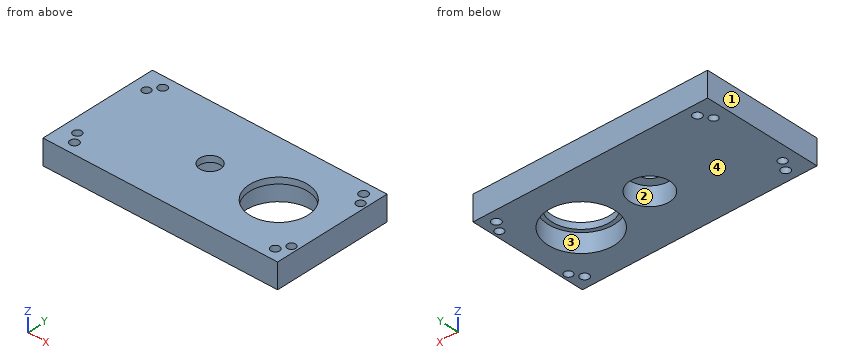
```python
from build123d import *

# Parameters (mm, degrees)
ESBO_O1_W                = 118
ESBO_O1_H                = 62
ESBO_O1_R                = 9.5
ESBO_O1_R_2              = 16
ESBO_O1_R_3              = 2
RESSALTO_EXTRUS_O1_DEPTH = 12
FURO_COM_FOLGA_DE_M51_D  = 4.2
RESSALTO_EXTRUS_O4_START = -3
ESBO_O17_R               = 9.5
RESSALTO_EXTRUS_O4_DEPTH = 3
ESBO_O18_W               = 118
ESBO_O18_H               = 62
ESBO_O18_W_2             = 112.82
ESBO_O18_H_2             = 57
CORTE_EXTRUS_O3_DEPTH    = 68.720011813
RESSALTO_EXTRUS_O5_START = -3
ESBO_O19_R               = 16
ESBO_O19_R_2             = 14
RESSALTO_EXTRUS_O5_DEPTH = 3
ESBO_O21_R               = 5
CORTE_EXTRUS_O4_DEPTH    = 10


with BuildPart() as part:
    # Esboço1 → Ressalto-extrusão1 (new body)
    with BuildSketch(Plane.XY):
        Rectangle(ESBO_O1_W, ESBO_O1_H)
        with Locations((-4.25, 0)):
            Circle(ESBO_O1_R, mode=Mode.SUBTRACT)
        with Locations((28.75, 0)):
            Circle(ESBO_O1_R_2, mode=Mode.SUBTRACT)
        with Locations((51.5, -18)):
            Circle(ESBO_O1_R_3, mode=Mode.SUBTRACT)
        with Locations((51.5, 18)):
            Circle(ESBO_O1_R_3, mode=Mode.SUBTRACT)
        with Locations((-51.5, -18)):
            Circle(ESBO_O1_R_3, mode=Mode.SUBTRACT)
        with Locations((-51.5, 18)):
            Circle(ESBO_O1_R_3, mode=Mode.SUBTRACT)
    extrude(amount=RESSALTO_EXTRUS_O1_DEPTH)

    # Furo com folga de M51 (through all)
    with Locations(Plane.XY.offset(12)):
        with Locations((-48.32, 23), (-48.32, -23), (48.32, -23), (48.32, 23)):
            Hole(FURO_COM_FOLGA_DE_M51_D / 2)

    # Esboço17 → Ressalto-extrusão4 (add)
    with BuildSketch(Plane.XY.offset(12).offset(RESSALTO_EXTRUS_O4_START)):
        with Locations((-4.25, 0)):
            Circle(ESBO_O17_R)
    extrude(amount=RESSALTO_EXTRUS_O4_DEPTH)

    # Esboço18 → Corte-extrusão3 (cut, through all)
    with BuildSketch(Plane.XY.offset(12)):
        Rectangle(ESBO_O18_W, ESBO_O18_H)
        with Locations((-1.91, 0)):
            Rectangle(ESBO_O18_W_2, ESBO_O18_H_2, mode=Mode.SUBTRACT)
    extrude(amount=-CORTE_EXTRUS_O3_DEPTH, mode=Mode.SUBTRACT)

    # Esboço19 → Ressalto-extrusão5 (add)
    with BuildSketch(Plane.XY.offset(12).offset(RESSALTO_EXTRUS_O5_START)):
        with Locations((28.75, 0)):
            Circle(ESBO_O19_R)
        with Locations((28.75, 0)):
            Circle(ESBO_O19_R_2, mode=Mode.SUBTRACT)
    extrude(amount=RESSALTO_EXTRUS_O5_DEPTH)

    # Esboço21 → Corte-extrusão4 (cut)
    with BuildSketch(Plane(origin=(0, 0, 9), x_dir=(-1, 0, 0), z_dir=(0, 0, -1))):
        with Locations((4.25, 0)):
            Circle(ESBO_O21_R)
    extrude(amount=-CORTE_EXTRUS_O4_DEPTH, mode=Mode.SUBTRACT)


solid = part.part
```
Geometry check sheet. Reference: the model listing, model coordinates, mm. Face numbers are marked on the shaded views. Coordinates: 2 decimals unless noted, no trailing zeros. Loops run counter-clockwise (first coordinate to the right, second up) from the corner with the lowest first, then second, coordinate; pieces in that order, holes last.
Item 1: Release check for a two-part mould opening along X. For the marked faces 1, 2, 3 and 4 record: released by +X, released by -X, zero draft, split by the parting line, or undercut.
Item 2: Sectioned sample at B-B, the plane y = 23. Record the boundary of the cut face in (x, z), then the cut area to 3 significant figures.
Item 3: Sectioned sample at A-A, the plane x = 51.5. Record the boundary of the cut face in (y, z), then the cut area to 3 significant figures.
Item 4: Go/stop test with a flat-tipped pin: pin 1 Ø4.5 at (x, y) = (51.5, -18) entering from -Z. Record where the tip stops, or that it passes through.
Item 5: Thickness scan on line 1 (Y direction, x = 48.32, z = 4.5); line 2 (Y direction, x = 28.75, z = 2.75); line 3 (Y direction, x = -4.25, z = 4.25). Record the ranges inside material, lowest first.
Item 6: Sectioned sample at D-D, the plane x = -4.25. Record the boundary of the cut face in (y, z).
Item 7: Sectioned sample at C-C, the plane z = 6. Count the separate pieces of the cut face and the enclosed holes in it, then the cut area to 3 significant figures.
Check result:
1. face 1: released by -X
1. face 2: undercut
1. face 3: undercut
1. face 4: zero draft
2. outline: (-58.32, 0) - (-50.42, 0) - (-50.42, 12) - (-58.32, 12) - close; (-46.22, 0) - (46.22, 0) - (46.22, 12) - (-46.22, 12) - close; (50.42, 0) - (54.5, 0) - (54.5, 12) - (50.42, 12) - close
2. area: 1,250 mm2
3. outline: (-28.5, 0) - (-20, 0) - (-20, 12) - (-28.5, 12) - close; (-16, 0) - (16, 0) - (16, 12) - (-16, 12) - close; (20, 0) - (28.5, 0) - (28.5, 12) - (20, 12) - close
3. area: 588 mm2
4. pin 1: stops at z = 0
5. line 1: y = -28.5 to -25.1, -20.9 to 20.9, 25.1 to 28.5
5. line 2: y = -28.5 to -16, 16 to 28.5
5. line 3: y = -28.5 to -9.5, 9.5 to 28.5
6. outline: (-28.5, 0) - (-9.5, 0) - (-9.5, 9) - (-5, 9) - (-5, 12) - (-28.5, 12) - close; (5, 9) - (9.5, 9) - (9.5, 0) - (28.5, 0) - (28.5, 12) - (5, 12) - close
7. separate pieces: 1
7. enclosed holes: 10
7. area: 5,240 mm2
